Read the model definition and answer for the solid it produces. Units are mm, in the model's axes. Give positions to 0.01 mm unless a question says otherwise; leave off trailing zeros. Loops run counter-clockwise (first coordinate to the right, second up) from the corner with the lowest first, then second, coordinate; pieces in that order, holes last.
(1) Find section C-C, the plane y = -0.85. Write down the section's boundary in (x, z), then the cut area to 3 significant figures.
(2) Find section B-B, the plane x = -11.5. Write down the section's boundary in (y, z), then the cut area to 3 significant figures.
(3) Straight lines are drawn through the part: probe 1 along Z at (x, y) = (0, -0.65); probe 2 along Z at (x, y) = (-39, -0.3); probe 3 along Z at (x, y) = (11, -0.8). For each, find the intervals that lie inside material, in ascending order.
(4) Find section A-A, the plane z = -31. Write down the section's boundary in (x, y).
(5) Determine the mould class of faces 1 (the face through (0.477, -0.507, -45.102)), 2 (the face through (-11.056, -0.493, -49.787)), 3 (the face through (22, -1, 38)) for opening direction X: pulls with the +X half, pulls with the -X half, needs draft (parallel to the pull), parting line crosses it, or undercut.
```python
from build123d import *

# Parameters (mm, degrees)
F0_R     = 51
F0_R_2   = 43.5
F1_DEPTH = 1
F2_D     = 4.4
F2_DEPTH = 2.5
F2_TIP   = 1.3218933619


with BuildPart() as f1:
    # F0 (on Front) → F1 (new body)
    with BuildSketch(Plane.XZ):
        Circle(F0_R)
        Circle(F0_R_2, mode=Mode.SUBTRACT)
    extrude(amount=F1_DEPTH)

    # F2
    with Locations(Plane(origin=(0, 0, 0), x_dir=(1, 0, 0), z_dir=(0, 1, 0))):
        with Locations((0, -47.25), (-47.25, 0), (0, 47.25), (47.25, 0)):
            Hole(F2_D / 2, depth=F2_DEPTH)
            with Locations((0, 0, -(F2_DEPTH + F2_TIP / 2))):  # 118° drill point
                Cone(0, F2_D / 2, F2_TIP, mode=Mode.SUBTRACT)


solid = f1.part
```
Entries:
1. outline: circle Ø102 at (0, 0); hole circle Ø4.4 at (-47.25, 0); hole circle Ø87 at (0, 0); hole circle Ø4.4 at (0, -47.25); hole circle Ø4.4 at (0, 47.25); hole circle Ø4.4 at (47.25, 0)
1. area: 2,170 mm2
2. outline: (-1, -49.69) - (0, -49.69) - (0, -41.95) - (-1, -41.95) - close; (-1, 41.95) - (0, 41.95) - (0, 49.69) - (-1, 49.69) - close
2. area: 15.5 mm2
3. probe 1: z = -51 to -49.45, -45.05 to -43.5, 43.5 to 45.05, 49.45 to 51
3. probe 2: z = -32.86 to -19.27, 19.27 to 32.86
3. probe 3: z = -49.8 to -42.09, 42.09 to 49.8
4. outline: (-40.5, -1) - (-30.52, -1) - (-30.52, 0) - (-40.5, 0) - close; (30.52, -1) - (40.5, -1) - (40.5, 0) - (30.52, 0) - close
5. face 1: undercut
5. face 2: parting line crosses it
5. face 3: needs draft
